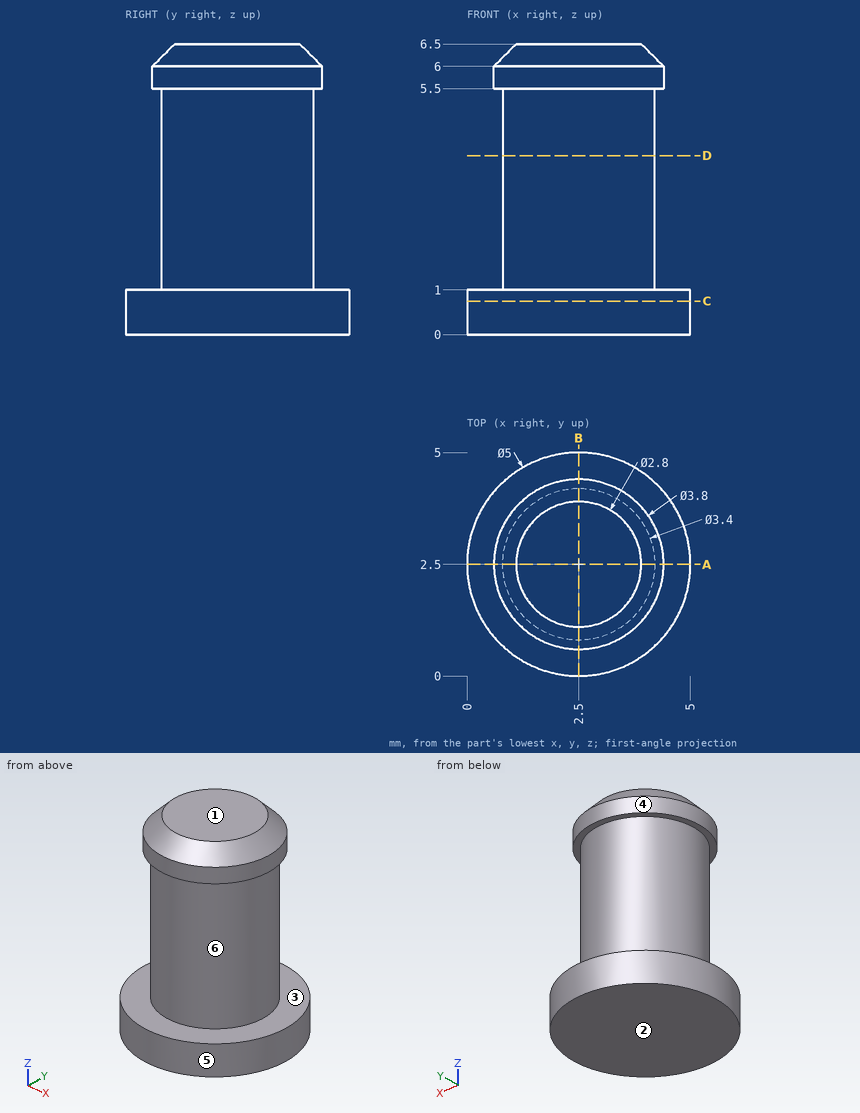
Geometry: see drawing. Coordinates: mm, zero at the bounding-box minimum. A direction names the side the tool comes from. Coordinates: 2 decimals unless noted, no trailing zeros. Order: outer loops, then holes, each group sorted by start corner. A loop starts at its lowest first (then second) coordinate and runs counter-clockwise, first axis right, second up. Notation, with made-up numbers: M 69.5,50 L 93.5,50 A15 cw 93.5,67 Z; hole C 56,15 d4. An arc over 180 degrees is marked long. Answer in a Markdown table with one row per item. Add a question column.
Q1. Line query: L1, parallel to Z at x = 0.65, y = 3.5; L2, parallel to X at y = 2.55, z = 5; L3, parallel to Y at x = 2.85, z = 2.5. Output: solid intervals per line, ascending.
Q2. Section query A-A on y = 2.5. Return the cut outline in (x, z), and give its area (4 significant figures).
Q3. Mould query, pull axis Z, two halves, no side actions, for the marked faces 1, 2 and 3. Classes: released by +Z, released by -Z, zero draft, split by the parting line, or undercut.
Q4. Section query C-C on z = 0.75. Return the cut outline in (x, y), and give its area (3 significant figures).
Q5. Section query D-D on z = 4. Return the cut outline in (x, y).
Q6. Contact query for flat-ended pins moving along their axis: P1, Ø1.9, axis at x = 3, y = 2, coming from the -Z side; P2, Ø2, axis at y = 1.5, z = 2.5, coming from the -X side; P3, Ø2, axis at x = 1, z = 5, coming from the +Y side. Output: stop coordinate, or through.
Q7. Reachability of the marked faces 4, 5 and 6 from +Z, -Z, +X, -X, +Y, -Y: full face, straight path, thin tool, end or side. Return the list, or none.
Completed:
| question | item | result |
|---|---|---|
| 1 | L1 | z = 0 to 1 |
| 1 | L2 | x = 0.8 to 4.2 |
| 1 | L3 | y = 0.84 to 4.16 |
| 2 | outline | M 0,0 L 5,0 L 5,1 L 4.2,1 L 4.2,5.5 L 4.4,5.5 L 4.4,6 L 3.9,6.5 L 1.1,6.5 L 0.6,6 L 0.6,5.5 L 0.8,5.5 L 0.8,1 L 0,1 Z |
| 2 | area | 23.85 mm2 |
| 3 | face 1 | released by +Z |
| 3 | face 2 | released by -Z |
| 3 | face 3 | undercut |
| 4 | outline | C 2.5,2.5 d5 |
| 4 | area | 19.6 mm2 |
| 5 | outline | C 2.5,2.5 d3.4 |
| 6 | P1 | stops at z = 0 |
| 6 | P2 | stops at x = 0.8 |
| 6 | P3 | stops at y = 4.29 |
| 7 | face 4 | +Z |
| 7 | face 5 | +Z, -Z |
| 7 | face 6 | none |
